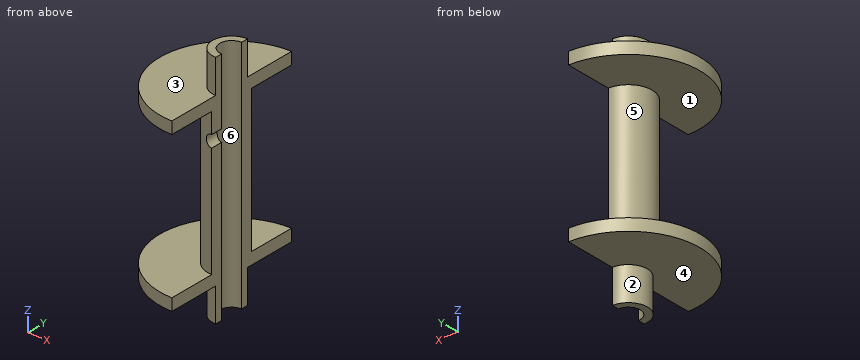
Autodesk Inventor part; units mm, degrees
ref_plane "YZ Plane" through (0, 0, 0) normal (1, 0, 0) x (0, 1, 0)
ref_plane "XZ Plane" through (0, 0, 0) normal (0, 1, 0) x (-1, 0, 0)
ref_plane "XY Plane" through (0, 0, 0) normal (0, 0, 1) x (1, 0, 0)
sketch "Sketch1" plane through (0, 0, 0) normal (0, 1, 0) x (-1, 0, 0)
  line L0 (0, 0) -> (2.5, 0)
  line L1 (2.5, 0) -> (2.5, -7)
  line L2 (0, 0) -> (4, 0)
  line L3 (4, 0) -> (4, -7)
  line L4 (2.5, -7) -> (4, -7)
  line L5 (4, -7) -> (4, 0)
  line L6 (4, 0) -> (2.5, 0)
  line L7 (2.5, 0) -> (2.5, -7)
  line L8 (2.5, -7) -> (15, -7)
  line L9 (15, -7) -> (15, -9.5)
  line L10 (15, -9.5) -> (2.5, -9.5)
  line L11 (2.5, -9.5) -> (2.5, -7)
  line L12 (2.5, -9.5) -> (5, -9.5)
  line L13 (5, -9.5) -> (5, -39.5)
  line L14 (5, -39.5) -> (2.5, -39.5)
  line L15 (2.5, -39.5) -> (2.5, -9.5)
  line L16 (5, -24.5) -> (-8.9655, -24.5)
  line L17 (0, -49) -> (2.5, -49)
  line L18 (2.5, -49) -> (2.5, -42)
  line L19 (0, -49) -> (4, -49)
  line L20 (4, -49) -> (4, -42)
  line L21 (2.5, -42) -> (4, -42)
  line L22 (4, -42) -> (4, -49)
  line L23 (4, -49) -> (2.5, -49)
  line L24 (2.5, -49) -> (2.5, -42)
  line L25 (2.5, -42) -> (15, -42)
  line L26 (15, -42) -> (15, -39.5)
  line L27 (15, -39.5) -> (2.5, -39.5)
  line L28 (2.5, -39.5) -> (2.5, -42)
  line L29 (2.5, -39.5) -> (5, -39.5)
  line L30 (0, 0) -> (0, -54.8818)
  dimension "d0" = 2.5
  dimension "d1" = 7
  dimension "d2" = 90
  dimension "d3" = 4
  dimension "d4" = 12.5
  dimension "d5" = 2.5
  dimension "d6" = 2.5
  dimension "d7" = 30
revolve "Revolution1" add sketch "Sketch1" angle 360 about axis through (0, 0, 0) along (0, 0, -1) contours L2 L3 L4 L1 | L4 L8 L9 L10 L11 | L16 L13 L14 L15 | L15 L10 L13 L16 | L14 L27 L26 L25 L21 L28 | L18 L21 L20 L19
sketch "Sketch2" plane through (0, 0, 0) normal (0, 1, 0) x (-1, 0, 0)
  line L0 (0, 0) -> (0, -15)
  line L1 (0, 0) -> (15, 0) construction
  circle A0 centre (0, -15) radius 1.25
  dimension "d9" = 15
  dimension "d10" = 90
  dimension "d11" = 2.5
extrude "Extrusion1" cut sketch "Sketch2" against normal blind 10
sketch "Sketch3" plane through (0, 0, 0) normal (0, 0, 1) x (1, 0, 0)
  circle A0 centre (0, 0) radius 4
  line L0 (0, 0) -> (24.6363, 0)
  line L1 (24.6363, 0) -> (24.6363, -18.6963)
  line L2 (24.6363, -18.6963) -> (0, -18.6963)
  line L3 (0, -18.6963) -> (0, 0)
  line L4 (0, 0) -> (27.3141, 0)
  line L5 (27.3141, 0) -> (27.3141, 19.6701)
  line L6 (27.3141, 19.6701) -> (0, 19.6701)
  line L7 (0, 19.6701) -> (0, 0)
extrude "Extrusion2" cut sketch "Sketch3" against normal blind 100 contours L0 L7 A0 | L0 L1 L2 L3 A0 | A0 L3 L0 | A0 L7 L6 L5 L4 L0
properties part number "spool"
The listing builds one solid part. Answer for the finished solid, in the listing's coordinates (mm). Face numbers are marked on the shaded views. A direction names the side the tool comes from. Round coordinates to 2 decimals unless told otherwise and drop trailing zeros. Order: outer loops, then holes, each group sorted by start corner. A loop starts at its lowest first (then second) coordinate and runs counter-clockwise, first axis right, second up. Notation, with made-up numbers: M 39,-21 L 57,-21 A10 cw 57,-14 Z; hole C 46,85 d1. An arc over 180 degrees is marked long. Answer in a Markdown table with one row per item. Add a question column.
1) Which of the six approach directions +Z, -Z, +X, -X, +Y, -Y give full straight-line access (tool end or side, diameter ignored) to the marked faces 1 and 2?
2) Flat-ended cylindrical pins translate along their axes: pin 1 Ø1 at (x, z) = (-6.5, -9.5) entering from +Y; pin 2 Ø10 at (y, z) = (6, -19.5) entering from -X; pin 3 Ø1 at (x, y) = (-2.5, -8) entering from -Z. Find the tip coordinate at first contact, or state that the pin passes through.
3) The part is cut by section D-D on x = -3.5. Determine the outline of the cut face in (y, z), plus the area to 3 significant figures.
4) Determine the mould class of the marked faces 3, 4, 5 and 6 for opening direction Z: pulls with the +Z half, pulls with the -Z half, needs draft (parallel to the pull), parting line crosses it, or undercut.
5) The part is cut by section C-C on y = 0. Determine the outline of the cut face in (x, z), plus the area to 4 significant figures.
6) The part is cut by section A-A on x = -8.75. Determine the outline of the cut face in (y, z), plus the area to 3 significant figures.
7) The part is cut by section B-B on y = 8. Determine the outline of the cut face in (x, z).
8) Consider line 1 along Z through (x, y) = (-4.5, 4.5); line 2 along X through (y, z) = (-2.25, -11.5); line 3 along Y through (x, z) = (-2.25, -36). Determine where each line is inside the solid, lowest interval first. Write a range as from..to.
Findings below:
| question | item | result |
|---|---|---|
| 1 | face 1 | -X |
| 1 | face 2 | -Z, -X |
| 2 | pin 1 | stops at y = 13.75 |
| 2 | pin 2 | stops at x = -4.9 |
| 2 | pin 3 | stops at z = -42 |
| 3 | outline | M -14.59,-42 L -1.94,-42 L -1.94,-49 L 1.94,-49 L 1.94,-42 L 14.59,-42 L 14.59,-39.5 L 3.57,-39.5 L 3.57,-9.5 L 14.59,-9.5 L 14.59,-7 L 1.94,-7 L 1.94,0 L -1.94,0 L -1.94,-7 L -14.59,-7 L -14.59,-9.5 L -3.57,-9.5 L -3.57,-39.5 L -14.59,-39.5 Z |
| 3 | area | 414 mm² |
| 4 | face 3 | pulls with the +Z half |
| 4 | face 4 | pulls with the -Z half |
| 4 | face 5 | undercut |
| 4 | face 6 | needs draft |
| 5 | outline | M -15,-42 L -4,-42 L -4,-49 L -2.5,-49 L -2.5,0 L -4,0 L -4,-7 L -15,-7 L -15,-9.5 L -5,-9.5 L -5,-39.5 L -15,-39.5 Z |
| 5 | area | 158.5 mm² |
| 6 | outline | M -12.18,-42 L 12.18,-42 L 12.18,-39.5 L -12.18,-39.5 Z; M -12.18,-9.5 L 12.18,-9.5 L 12.18,-7 L -12.18,-7 Z |
| 6 | area | 122 mm² |
| 7 | outline | M -12.69,-42 L 0,-42 L 0,-39.5 L -12.69,-39.5 Z; M -12.69,-9.5 L 0,-9.5 L 0,-7 L -12.69,-7 Z |
| 8 | line 1 | z = -42..-39.5, -9.5..-7 |
| 8 | line 2 | x = -4.47..-1.09 |
| 8 | line 3 | y = -4.47..-1.09, 1.09..4.47 |
